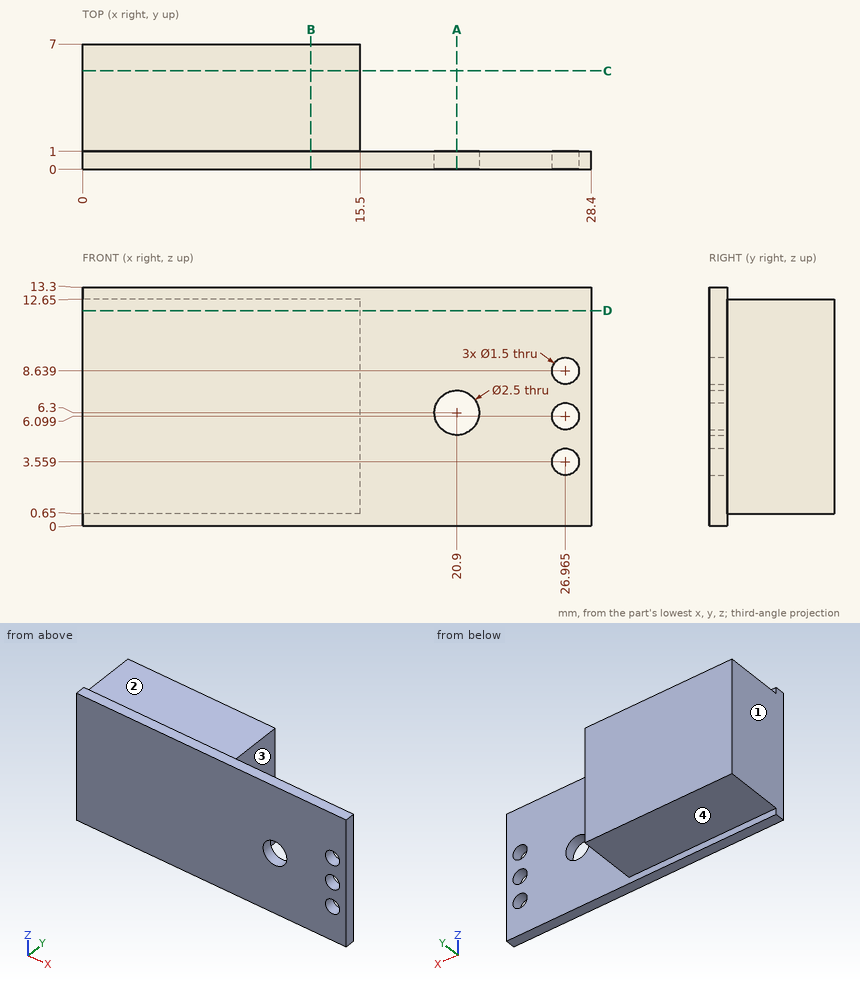
Input: dimensioned drawing with shaded views. Units: mm. Origin: part minimum x, y, z. A direction names the side the tool comes from. Coordinates: 2 decimals unless noted, no trailing zeros. Order: outer loops, then holes, each group sorted by start corner. A loop starts at its lowest first (then second) coordinate and runs counter-clockwise, first axis right, second up.
1. Cut plane A-A, the plane x = 20.9. Return loops of the section in (y, z), plus the area to 3 significant figures.
Checked values:
outline: (0, 0) - (1, 0) - (1, 5.05) - (0, 5.05) - close; (0, 7.55) - (1, 7.55) - (1, 13.3) - (0, 13.3) - close
area: 10.8 mm2
2. Cut plane D-D, the plane z = 12. Return loops of the section in (x, y), plus the area to 3 significant figures.
Checked values:
outline: (0, 0) - (28.4, 0) - (28.4, 1) - (15.5, 1) - (15.5, 7) - (0, 7) - close
area: 121 mm2
3. Cut plane B-B, the plane x = 12.75. Return loops of the section in (y, z), plus the area to 3 significant figures.
Checked values:
outline: (0, 0) - (1, 0) - (1, 0.65) - (7, 0.65) - (7, 12.65) - (1, 12.65) - (1, 13.3) - (0, 13.3) - close
area: 85.3 mm2
4. Access query for the marked faces 1, 2, 3 and 4. Directions: +Z, -Z, +X, -X, +Y, -Y. A direction counts if a zero-diameter tool reaches every point of the face in a straight line with its end or side. Return the directions, or none.
Checked values:
face 1: +Z, -Z, -X, +Y, -Y
face 2: +Z, +X, -X, +Y
face 3: +Z, -Z, +X, +Y
face 4: -Z, +X, -X, +Y
5. Ray query, line 1 along Z through (x, y) = (20.9, 0.55); line 2 along X through (y, z) = (1.75, 8.5); line 3 along X through (y, z) = (0.5, 6.25). Return the intervals inside material, ascending.
Checked values:
line 1: z = 0 to 5.05, 7.55 to 13.3
line 2: x = 0 to 15.5
line 3: x = 0 to 19.65, 22.15 to 26.23, 27.7 to 28.4
6. Contact query for flat-ended pins moving along their axis: P1, Ø2.5, axis at x = 26.97, z = 3.56, coming from the +Y side; P2, Ø3, axis at y = 6, z = 10, coming from the +X side; P3, Ø4, axis at x = 12, y = 5.5, coming from the -Z side. Output: stop coordinate, or through.
Checked values:
P1: stops at y = 1
P2: stops at x = 15.5
P3: stops at z = 0.65
7. Cut plane C-C, the plane y = 5.5. Return loops of the section in (x, z).
Checked values:
outline: (0, 0.65) - (15.5, 0.65) - (15.5, 12.65) - (0, 12.65) - close
